from build123d import *

# Parameters (mm, degrees)
SKETCH1_R                                = 165.1
SKETCH1_R_2                              = 44.577
SKETCH1_R_3                              = 17.4625
BOSS_EXTRUDE1_DEPTH                      = 12.7
CBORE_FOR_1_4_HEX_HEAD_BOLT1_D           = 6.5786
CBORE_FOR_1_4_HEX_HEAD_BOLT1_CBORE_D     = 12.7
CBORE_FOR_1_4_HEX_HEAD_BOLT1_CBORE_DEPTH = 3.81


with BuildPart() as part:
    # Sketch1 → Boss-Extrude1 (new body)
    with BuildSketch(Plane.XY):
        with Locations((0, -8.643025507)):
            Circle(SKETCH1_R)
        with Locations((0, -114.3)):
            Circle(SKETCH1_R_2, mode=Mode.SUBTRACT)
        Circle(SKETCH1_R_3, mode=Mode.SUBTRACT)
    extrude(amount=BOSS_EXTRUDE1_DEPTH)

    # CBORE for 1/4 Hex Head Bolt1 (through all)
    with Locations(Plane(origin=(0, 0, 0), x_dir=(-1, 0, 0), z_dir=(0, 0, -1))):
        with Locations((-40.005, 49.2125), (40.005, 49.2125), (40.005, -49.2125), (-40.005, -49.2125)):
            CounterBoreHole(CBORE_FOR_1_4_HEX_HEAD_BOLT1_D / 2, CBORE_FOR_1_4_HEX_HEAD_BOLT1_CBORE_D / 2, CBORE_FOR_1_4_HEX_HEAD_BOLT1_CBORE_DEPTH)


solid = part.part
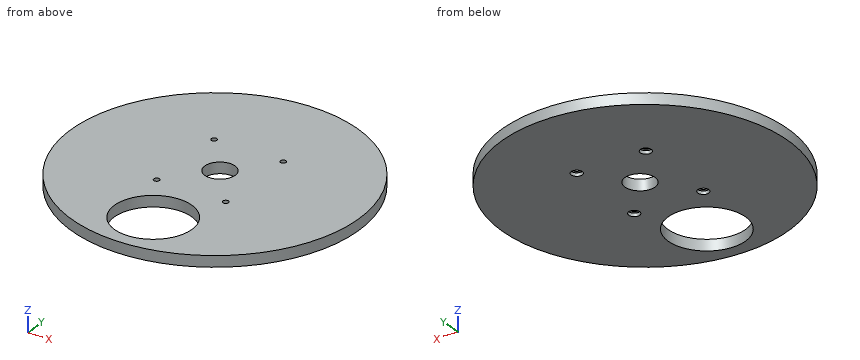
Verification items for the finished model (mm, model axes). Coordinates: 2 decimals unless noted, no trailing zeros. Loops run counter-clockwise (first coordinate to the right, second up) from the corner with the lowest first, then second, coordinate; pieces in that order, holes last. Notation, with made-up numbers: (55, 65.5) -> (113, 65.5) arc R25 cw to (113, 85.5) -> close; hole circle Ø4 at (-34.75, 78.5). An arc over 180 degrees is marked (long way). Answer as CSV lines item,"result".
1) Cross-section at C-C, the plane z = 6. Record the cut outline in (x, y) (1 decimal).
Found:
outline,"circle Ø330.2 at (0, -8.6); hole circle Ø89.2 at (0, -114.3); hole circle Ø6.6 at (-40, -49.2); hole circle Ø6.6 at (-40, 49.2); hole circle Ø34.9 at (0, 0); hole circle Ø6.6 at (40, -49.2); hole circle Ø6.6 at (40, 49.2)"
2) Cross-section at A-A, the plane x = 0. Record the cut outline in (y, z).
Found:
outline,"(-173.74, 0) -> (-158.88, 0) -> (-158.88, 12.7) -> (-173.74, 12.7) -> close; (-69.72, 0) -> (-17.46, 0) -> (-17.46, 12.7) -> (-69.72, 12.7) -> close; (17.46, 0) -> (156.46, 0) -> (156.46, 12.7) -> (17.46, 12.7) -> close"
3) Depth check by flat-ended pin: pin 1 (4 mm diameter, centred on x = 39, y = 47.5, fed in from -Z); pin 2 (6 mm diameter, centred on x = -36.5, z = 10.5, fed in from -Y); pin 3 (3 mm diameter, centred on x = 92.5, z = 5, fed in from -Y). Enter the tip coordinate at first touch or a pass-through.
Found:
pin 1,"stops at z = 3.81"
pin 2,"stops at y = -170.31"
pin 3,"stops at y = -146.4"
4) Cross-section at B-B, the plane y = -127. Record the cut outline in (x, z), then the cut area to 3 significant figures.
Found:
outline,"(-115.11, 0) -> (-42.73, 0) -> (-42.73, 12.7) -> (-115.11, 12.7) -> close; (42.73, 0) -> (115.11, 0) -> (115.11, 12.7) -> (42.73, 12.7) -> close"
area,"1,840 mm2"
5) Thickness scan on L1, parallel to Y at x = 0, z = 8.5; L2, parallel to Y at x = -35, z = 1; L3, parallel to Y at x = -5.5, z = 0.75. Record the ranges inside material, lowest first. Write a range as from..to.
Found:
L1,"y = -173.74..-158.88, -69.72..-17.46, 17.46..156.46"
L2,"y = -169.99..-141.91, -86.69..-53.12, -45.3..45.3, 53.12..152.7"
L3,"y = -173.65..-158.54, -70.06..-16.57, 16.57..156.37"
6) Cross-section at D-D, the plane y = 0. Record the cut outline in (x, z).
Found:
outline,"(-164.87, 0) -> (-17.46, 0) -> (-17.46, 12.7) -> (-164.87, 12.7) -> close; (17.46, 0) -> (164.87, 0) -> (164.87, 12.7) -> (17.46, 12.7) -> close"
